```python
from build123d import *

# Parameters (mm, degrees)
BOSS_EXTRUDE1_DEPTH     = 40.2
CUT_EXTRUDE1_DEPTH      = 102.00019802
CUT_EXTRUDE1_DEPTH_BACK = 102.00019802
SKETCH2_R               = 5.5
FILLET1_R               = 15
CUT_EXTRUDE2_DEPTH      = 100.458735162
CUT_EXTRUDE2_DEPTH_BACK = 100.458735162
SKETCH4_R               = 1.28125
SKETCH4_R_2             = 1.035449613


with BuildPart() as part:
    # Sketch1 → Boss-Extrude1 (new body)
    with BuildSketch(Plane(origin=(0, 0, 0), x_dir=(1, 0, 0), z_dir=(0, 1, 0))):
        Polygon((0, 3), (0, 0), (76, 0), (76, 53), (0, 53), (0, 50), (73, 50), (73, 3), align=None)
    extrude(amount=BOSS_EXTRUDE1_DEPTH)

    # Sketch2 → Cut-Extrude1 (cut, two sides: drawn at the far end of the back side and taken through both)
    with BuildSketch(Plane.XY.offset(-CUT_EXTRUDE1_DEPTH_BACK)):
        with Locations((15.5, 20.1)):
            Circle(SKETCH2_R)
    extrude(amount=CUT_EXTRUDE1_DEPTH + CUT_EXTRUDE1_DEPTH_BACK, mode=Mode.SUBTRACT)

    # Fillet1
    fillet1_edges = [part.edges().sort_by_distance(p)[0] for p in [
        (0, 0, -1.5),
        (0, 40.2, -1.5),
        (0, 40.2, -51.5),
        (0, 0, -51.5),
    ]]
    fillet(fillet1_edges, radius=FILLET1_R)

    # Sketch4 → Cut-Extrude2 (cut, two sides: drawn at the far end of the back side and taken through both)
    with BuildSketch(Plane.XY.offset(-50).offset(-CUT_EXTRUDE2_DEPTH_BACK)):
        with Locations((15.746359238, 9.102759113)):
            Circle(SKETCH4_R)
        with Locations((7.897978682, 12.149574107)):
            Circle(SKETCH4_R)
        with Locations((4.502759113, 19.607840375)):
            Circle(SKETCH4_R_2)
        with Locations((7.549574107, 27.702021318)):
            Circle(SKETCH4_R)
        with Locations((23.450425893, 12.497978682)):
            Circle(SKETCH4_R)
        with Locations((15.253640762, 31.097240887)):
            Circle(SKETCH4_R)
        with Locations((23.102021318, 28.050425893)):
            Circle(SKETCH4_R)
        with Locations((26.497240887, 20.346359238)):
            Circle(SKETCH4_R)
    extrude(amount=CUT_EXTRUDE2_DEPTH + CUT_EXTRUDE2_DEPTH_BACK, mode=Mode.SUBTRACT)


solid = part.part
```
CAD build for the part. Positions are in the model's coordinates, mm. A direction names the side the tool comes from. Coordinates: 2 decimals unless noted, no trailing zeros. Order: outer loops, then holes, each group sorted by start corner. A loop starts at its lowest first (then second) coordinate and runs counter-clockwise, first axis right, second up.
(1) Saw through at C-C, the plane z = -9. Write the cut outline in (x, y), and give its area (3 significant figures).
Solution:
outline: (73, 0) - (76, 0) - (76, 40.2) - (73, 40.2) - close
area: 121 mm2
(2) Which spindle directions (+Z, -Z, +X, -X, +Y, -Y) get a long thin tool onto all of the face, cutting with end or side? Do faces 1 (the face through (36, 20, -50)), 2 (the face through (0, 20, -52)). Say none if no direction does.
Solution:
face 1: -X, +Y, -Y
face 2: +Z, -Z, -X, +Y, -Y
(3) Saw through at B-B, the plane y = 23.5. Write the cut outline in (x, z), and give its area (3 significant figures).
Solution:
outline: (0, -53) - (11.18, -53) - (11.18, -50) - (0, -50) - close; (0, -3) - (11.18, -3) - (11.18, 0) - (0, 0) - close; (19.82, -53) - (76, -53) - (76, 0) - (19.82, 0) - (19.82, -3) - (73, -3) - (73, -50) - (19.82, -50) - close
area: 545 mm2
(4) Drill centre lines: L1, parallel to Z at x = 7, y = 3; L2, parallel to X at y = 22.5, z = -39.5. Where is each one in solid material? Low to high.
Solution:
L1: z = -53 to -50, -3 to 0
L2: x = 73 to 76
(5) Saw through at A-A, the plane x = 48.5. Write the cut outline in (y, z).
Solution:
outline: (0, -53) - (40.2, -53) - (40.2, -50) - (0, -50) - close; (0, -3) - (40.2, -3) - (40.2, 0) - (0, 0) - close
(6) Pin check, flat tips, straight feed: pin 1 Ø2 at (x, y) = (26.5, 20.35) entering from +Z; pin 2 Ø2 at (y, z) = (19.5, -21) entering from -X. Stop position of each tip, or through.
Solution:
pin 1: passes through
pin 2: stops at x = 73
(7) Mould opens along Z. For faces 3 (the face through (4.51, 35.92, -51.48)), 4 (the face through (73, 20, -27)) say: released by +Z, released by -Z, zero draft, split by the parting line, or undercut.
Solution:
face 3: zero draft
face 4: undercut
